Part model, mm, in its own coordinate system. Face numbers are marked on the shaded views. A direction names the side the tool comes from. Round coordinates to 2 decimals unless told otherwise and drop trailing zeros. Order: outer loops, then holes, each group sorted by start corner. A loop starts at its lowest first (then second) coordinate and runs counter-clockwise, first axis right, second up. Notation, with made-up numbers: (31, 27.25) - (40, 27.25) arc R9 ccw to (40, 41.25) - close; hole circle Ø5 at (-34.5, -28). An arc over 180 degrees is marked (long way). Answer as a JSON object with one key per item and string values.
```python
from build123d import *

# Parameters (mm, degrees)
CYLINDER006_R               = 2
CYLINDER006_DEPTH           = 6
CYLINDER006_PITCH_ANGLE     = -90
CYLINDER006_PLACEMENT_ANGLE = -30.000033
CYLINDER007_R               = 2
CYLINDER007_DEPTH           = 6
CYLINDER007_PITCH_ANGLE     = -90
CYLINDER007_PLACEMENT_ANGLE = -30.000033
BOX012_W                    = 6
BOX012_H                    = 4
BOX012_DEPTH                = 9
BOX012_PLACEMENT_ANGLE      = 30


with BuildPart() as cylinder006:
    # Cylinder006 → Cylinder006 (new body)
    with BuildSketch(Plane.XY):
        Circle(CYLINDER006_R)
    extrude(amount=CYLINDER006_DEPTH)


with BuildPart() as cylinder006_1:
    # Cylinder006 pitch: moved
    add(cylinder006.part.rotate(Axis((0, 0, 0), (0, 1, 0)), CYLINDER006_PITCH_ANGLE))


with BuildPart() as cylinder006_2:
    # Cylinder006 placement: moved
    add(cylinder006_1.part.moved(Location((12.102594, -9.316468, -1e-06))).rotate(Axis((12.102594, -9.316468, -1e-06), (0, 0, 1)), CYLINDER006_PLACEMENT_ANGLE))


with BuildPart() as cylinder007:
    # Cylinder007 → Cylinder007 (new body)
    with BuildSketch(Plane.XY):
        Circle(CYLINDER007_R)
    extrude(amount=CYLINDER007_DEPTH)


with BuildPart() as cylinder007_1:
    # Cylinder007 pitch: moved
    add(cylinder007.part.rotate(Axis((0, 0, 0), (0, 1, 0)), CYLINDER007_PITCH_ANGLE))


with BuildPart() as cylinder007_2:
    # Cylinder007 placement: moved
    add(cylinder007_1.part.moved(Location((12.15259, -9.229864, 8.999999))).rotate(Axis((12.15259, -9.229864, 8.999999), (0, 0, 1)), CYLINDER007_PLACEMENT_ANGLE))


with BuildPart() as fusion011:
    # Box012 → Box012 (new body)
    with BuildSketch(Plane.XY):
        with Locations((3, 2)):
            Rectangle(BOX012_W, BOX012_H)
    extrude(amount=BOX012_DEPTH)


with BuildPart() as fusion011_1:
    # Box012 placement: moved
    add(fusion011.part.moved(Location((5.915496, -8.034102, 0))).rotate(Axis((5.915496, -8.034102, 0), (0, 0, -1)), BOX012_PLACEMENT_ANGLE))

    # Fusion011: union Cylinder006, Cylinder007
    add(cylinder006_2.part)
    add(cylinder007_2.part)


solid = fusion011_1.part
```
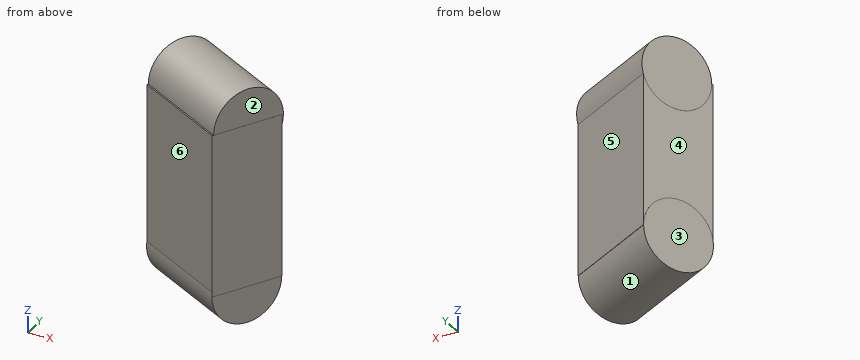
Item 1: Cut at B-B (z = -0.25). Write the cut outline in (x, y), plus the area to 3 significant figures.
Taken from the geometry:
{"outline": "(5.91, -8.03) - (11.11, -11.03) - (13.09, -7.6) - (7.9, -4.6) - close", "area": "23.8 mm2"}
Item 2: Two-plate mould, pull along X, no slides. Class the marked faces 1, 2 and 3: pulls with the +X half, pulls with the -X half, needs draft (parallel to the pull), parting line crosses it, or undercut.
Taken from the geometry:
{"face 1": "parting line crosses it", "face 2": "pulls with the +X half", "face 3": "pulls with the -X half"}
Item 3: Tool access for the marked faces 4, 5 and 6: list every direction of +Z, -Z, +X, -X, +Y, -Y with a clear straight run to the whole face (end or side of a thin tool).
Taken from the geometry:
{"face 4": "+Z, -Z, -X, +Y", "face 5": "-Z, +X, +Y", "face 6": "+Z, -X, -Y"}
Item 4: Cut at A-A (z = 6.5). Write the cut outline in (x, y), plus the area to 3 significant figures.
Taken from the geometry:
{"outline": "(5.92, -8.03) - (11.11, -11.03) - (13.11, -7.57) - (7.92, -4.57) - close", "area": "24.0 mm2"}
Item 5: Probe L1, parallel to X at y = -6.5, z = 2.25; L2, parallel to X at y = -8.75, z = 7.75; L3, parallel to Z at x = 11, y = -8. List the from-to ranges inside material, lowest first. Write a range as from..to.
Taken from the geometry:
{"L1": "6.8..11.26", "L2": "7.16..12.43", "L3": "-1.91..10.94"}
Item 6: Drop flat-ended pins along their axis: P1, Ø2, axis at x = 8, z = 9, coming from the -Y side; P2, Ø3, axis at x = 6.5, z = 0, coming from the -Y side; P3, Ø3, axis at y = -7.5, z = 4.5, coming from the -X side. Give the stop position or say it passes through.
Taken from the geometry:
{"P1": "y = -9.81", "P2": "y = -9.26", "P3": "x = 5.92"}
